Autodesk Inventor part; units mm, degrees
ref_plane "YZ Plane" through (0, 0, 0) normal (1, 0, 0) x (0, 1, 0)
ref_plane "XZ Plane" through (0, 0, 0) normal (0, 1, 0) x (-1, 0, 0)
ref_plane "XY Plane" through (0, 0, 0) normal (0, 0, 1) x (1, 0, 0)
sketch "Sketch2" plane through (0, 0, 0) normal (0, 0, 1) x (1, 0, 0)
  line L0 (-25, 75) -> (25, 75)
  line L1 (25, 75) -> (25, -75)
  line L2 (25, -75) -> (-25, -75)
  line L3 (-25, -75) -> (-25, 75)
  line L4 (-25, 75) -> (25, -75) construction
  line L5 (25, 75) -> (-25, -75) construction
  point P0 (0, 0)
  dimension "d0" = 50
  dimension "d1" = 150
extrude "Extrusion1" add sketch "Sketch2" along normal blind 6
fillet "Fillet1" radius 2 4 edges at (25, 75, 3) (-25, 75, 3) (25, -75, 3) (-25, -75, 3)
sketch "Sketch3" plane through (0, 0, 6) normal (0, 0, 1) x (1, 0, 0)
  line L0 (23, 75) -> (-23, 75)
  point P0 (0, 0)
  point P1 (0, 38.6)
  point P2 (0, 75)
  dimension "d5" = 36.4
hole "Hole1" at (0, 38.6, 6) direction (0, 0, -1) diameter 10.5 end through all
sketch "Sketch4" plane through (0, 0, 6) normal (0, 0, 1) x (1, 0, 0)
  line L0 (-23, -75) -> (23, -75)
  point P0 (0, 0)
  point P1 (0, -55.449)
  point P2 (0, -35.449)
  dimension "d13" = 20
  dimension "d14" = 39.551
hole "Hole2" at (0, -55.449, 6) at (0, -35.449, 6) direction (0, 0, -1) diameter 5.4 end through all
properties part number "Columna"
Work out the finished part from the listing and answer in its coordinate system (mm). Coordinates: 2 decimals unless noted, no trailing zeros. Write each loop counter-clockwise with the first axis right and the second up, starting at its lowest first coordinate (ties: lowest second). Pieces come first, ordered by that corner, then holes.
Q1. Determine the mould class of faces 1 (the face through (-0.12, -52.75, 2.96)), 2 (the face through (-0.811, -38.024, 2.958)), 3 (the face through (-25, -1, 3)), 4 (the face through (0, 75, 3)) for opening direction Y: released by +Y, released by -Y, zero draft, split by the parting line, or undercut.
Q2. A cutting plane is placed at B-B, the plane x = 0. Give the vertices of the cut face in (y, z), then the cut area to 3 significant figures.
Q3. A cutting plane is placed at C-C, the plane y = 38.6. Give the vertices of the cut face in (x, z).
Q4. Find the intervals of material crossed by line 1 (Y direction, x = 0, z = 4.2); line 2 (X direction, y = 38.6, z = 3.8); line 3 (Y direction, x = 2, z = 5.2), in increasing order.
Q5. This flat-tipped pin is pushed along its axis until it touches: pin 1 Ø3 at (x, y) = (0, -55.449) entering from -Z. Where does it stop, or does it pass through?
Q6. A cutting plane is placed at A-A, the plane z = 2.8. Give the vertices of the cut face in (x, y), then the cut area to 3 significant figures.
Findings below:
1. face 1: undercut
1. face 2: undercut
1. face 3: zero draft
1. face 4: released by +Y
2. outline: (-75, 0) - (-58.15, 0) - (-58.15, 6) - (-75, 6) - close; (-52.75, 0) - (-38.15, 0) - (-38.15, 6) - (-52.75, 6) - close; (-32.75, 0) - (33.35, 0) - (33.35, 6) - (-32.75, 6) - close; (43.85, 0) - (75, 0) - (75, 6) - (43.85, 6) - close
2. area: 772 mm2
3. outline: (-25, 0) - (-5.25, 0) - (-5.25, 6) - (-25, 6) - close; (5.25, 0) - (25, 0) - (25, 6) - (5.25, 6) - close
4. line 1: y = -75 to -58.15, -52.75 to -38.15, -32.75 to 33.35, 43.85 to 75
4. line 2: x = -25 to -5.25, 5.25 to 25
4. line 3: y = -75 to -57.26, -53.64 to -37.26, -33.64 to 33.75, 43.45 to 75
5. pin 1: passes through
6. outline: (-25, -73) arc R2 ccw to (-23, -75) - (23, -75) arc R2 ccw to (25, -73) - (25, 73) arc R2 ccw to (23, 75) - (-23, 75) arc R2 ccw to (-25, 73) - close; hole circle Ø10.5 at (0, 38.6); hole circle Ø5.4 at (0, -55.45); hole circle Ø5.4 at (0, -35.45)
6. area: 7,360 mm2
